The listing builds one solid part. Answer for the finished solid, in the listing's coordinates (mm). Face numbers are marked on the shaded views. Give positions to 0.01 mm unless a question says otherwise; leave off trailing zeros. Use one line per item in the form item = value. Start each with the question number.
1. The mould has two halves that part along Y. Classify the marked faces 1 and 2: released by +Y, released by -Y, zero draft, split by the parting line, or undercut.
2. Each of these flat-tipped pins is pushed along its axis until it touches: pin 1 Ø3 at (x, y) = (-129.5, 373) entering from +Z; pin 2 Ø5 at (x, z) = (344, 16) entering from +Y; pin 3 Ø10 at (y, z) = (-220.5, 43.5) entering from +X. Where does it stop, or does it pass through?
3. Straight lines are drawn through the part: line 1 (Y direction, x = -4, z = 45); line 2 (Y direction, x = 0, z = 49); line 3 (X direction, y = 37, z = 18.5). For each, find the intervals that lie inside material, in ascending order. Write a range as from..to.
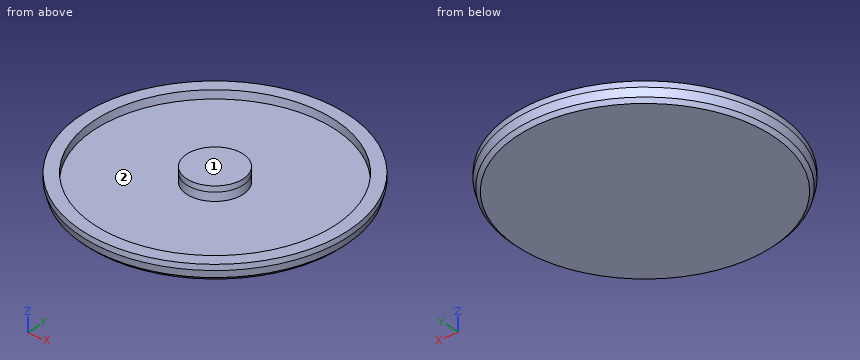
from build123d import *

# Parameters (mm, degrees)
SKETCH2_R           = 470
BOSS_EXTRUDE1_DEPTH = 60
BOSS_EXTRUDE2_START = -60
SKETCH3_R           = 100
BOSS_EXTRUDE2_DEPTH = 80
SKETCH4_R           = 425
SKETCH4_R_2         = 100
CUT_EXTRUDE2_DEPTH  = 30
CHAMFER2_SIZE       = 20
CHAMFER8_SIZE       = 20
CHAMFER8_SIZE2      = 10.352761804


with BuildPart() as part:
    # Sketch2 → Boss-Extrude1 (new body)
    with BuildSketch(Plane.XY):
        Circle(SKETCH2_R)
    extrude(amount=BOSS_EXTRUDE1_DEPTH)

    # Sketch3 → Boss-Extrude2 (add)
    with BuildSketch(Plane.XY.offset(60).offset(BOSS_EXTRUDE2_START)):
        Circle(SKETCH3_R)
    extrude(amount=BOSS_EXTRUDE2_DEPTH)

    # Sketch4 → Cut-Extrude2 (cut)
    with BuildSketch(Plane.XY.offset(60)):
        Circle(SKETCH4_R)
        Circle(SKETCH4_R_2, mode=Mode.SUBTRACT)
    extrude(amount=-CUT_EXTRUDE2_DEPTH, mode=Mode.SUBTRACT)

    # Chamfer2
    chamfer2_edges = [part.edges().sort_by_distance(p)[0] for p in [
        (-470, 0, 0),
    ]]
    chamfer(chamfer2_edges, length=CHAMFER2_SIZE)

    # Chamfer8
    chamfer8_edges = [part.edges().sort_by_distance(p)[0] for p in [
        (-470, 0, 20),
    ]]
    chamfer8_side = [part.faces().sort_by_distance(p)[0] for p in [
        (-470, 0, 40),
    ]]
    chamfer(chamfer8_edges, length=CHAMFER8_SIZE, length2=CHAMFER8_SIZE2, reference=chamfer8_side[0])


solid = part.part
Derived:
q1.face_1 = zero draft
q1.face_2 = undercut
q2.pin_1 = 30
q2.pin_2 = 313.66
q2.pin_3 = 417.68
q3.line_1 = -469.98..-424.98, -99.92..99.92, 424.98..469.98
q3.line_2 = -470..-425, -100..100, 425..470
q3.line_3 = -462.76..462.76
